The figure shows three views and two pictorial views of one solid part (mm, origin at its lowest corner). Answer the questions. A direction names the side the tool comes from. Round coordinates to 2 decimals unless told otherwise and drop trailing zeros. Order: outer loops, then holes, each group sorted by start corner. A loop starts at its lowest first (then second) coordinate and runs counter-clockwise, first axis right, second up. Notation, with made-up numbers: (43, 18) - (58, 18) arc R23 ccw to (58, 35) - close; hole circle Ø5 at (6.25, 55.5). An arc over 180 degrees is marked (long way). Answer in a Markdown table with one row per item.
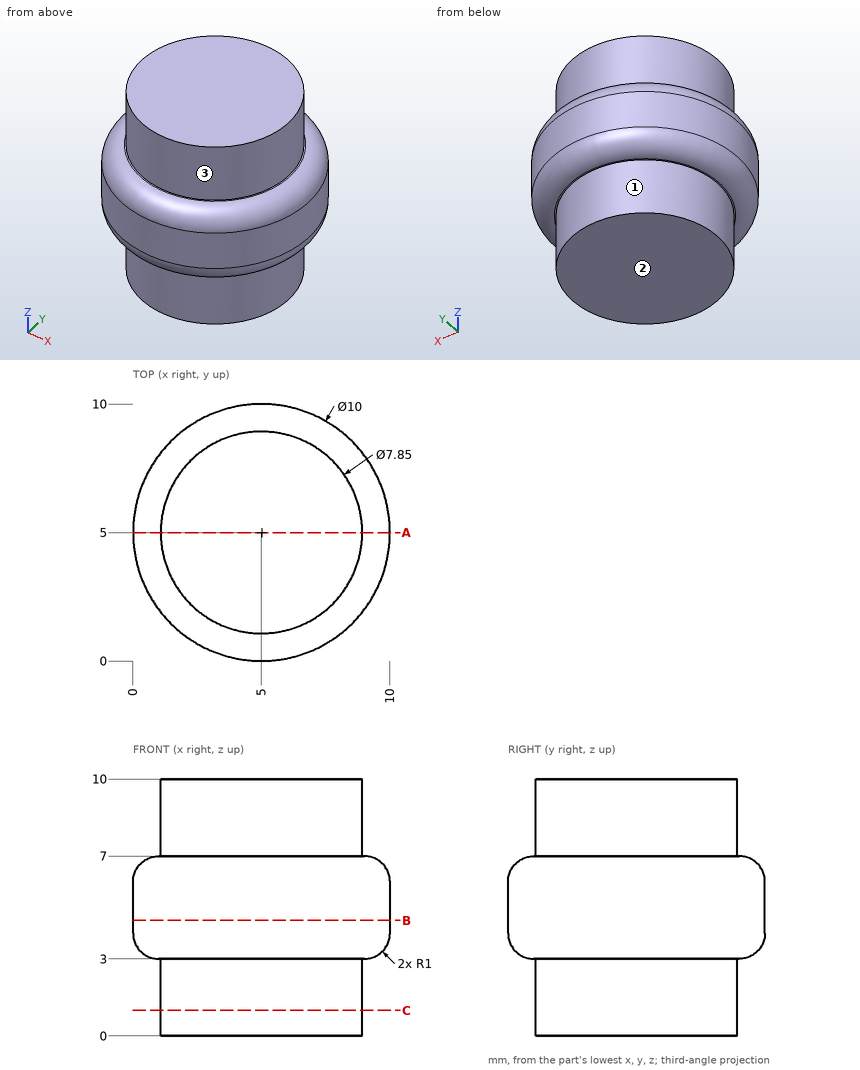
1) Find section A-A, the plane y = 5. Give the vertices of the cut face in (x, z) (3 decimals), then the cut area to 3 significant figures.
Filled in:
| item | result |
|---|---|
| outline | (0, 4) arc R1 ccw to (1, 3) - (1.075, 3) - (1.075, 0) - (8.925, 0) - (8.925, 3) - (9, 3) arc R1 ccw to (10, 4) - (10, 6) arc R1 ccw to (9, 7) - (8.925, 7) - (8.925, 10) - (1.075, 10) - (1.075, 7) - (1, 7) arc R1 ccw to (0, 6) - close |
| area | 86.2 mm^2 |
2) Each of these flat-tipped pins is pushed along its axis until it touches: pin 1 (1.5 mm diameter, centred on x = 8, z = 1.5, fed in from +Y); pin 2 (1.5 mm diameter, centred on x = 3, z = 3.5, fed in from +Y); pin 3 (1 mm diameter, centred on x = 7.5, z = 1.5, fed in from +Y). Where does it stop, or does it pass through?
Filled in:
| item | result |
|---|---|
| pin 1 | stops at y = 8.22 |
| pin 2 | stops at y = 9.81 |
| pin 3 | stops at y = 8.38 |
3) Find section B-B, the plane z = 4.5. Give the vertices of the cut face in (x, y).
Filled in:
| item | result |
|---|---|
| outline | circle Ø10 at (5, 5) |
4) Find section C-C, the plane z = 1. Give the vertices of the cut face in (x, y) (3 decimals), then the cut area to 3 significant figures.
Filled in:
| item | result |
|---|---|
| outline | circle Ø7.85 at (5, 5) |
| area | 48.4 mm^2 |
5) Which of the six approach directions +Z, -Z, +X, -X, +Y, -Y give full straight-line access (tool end or side, diameter ignored) to the marked faces 1, 2 and 3?
Filled in:
| item | result |
|---|---|
| face 1 | -Z |
| face 2 | -Z, +X, -X, +Y, -Y |
| face 3 | +Z |
6) Find the intervals of material crossed by probe 1 along X at (y, z) = (8, 6.5); probe 2 along Z at (x, y) = (1.5, 2); probe 3 along Z at (x, y) = (4.75, 9.5), in increasing order. Write a range as from..to.
Filled in:
| item | result |
|---|---|
| probe 1 | x = 1.17..8.83 |
| probe 2 | z = 3.21..6.79 |
| probe 3 | z = 3.14..6.86 |
